from build123d import *

# Parameters (mm, degrees)
SKETCH1_W           = 180
SKETCH1_H           = 165
BOSS_EXTRUDE1_DEPTH = 5
SKETCH2_W           = 4
SKETCH2_H           = 40
CUT_EXTRUDE1_DEPTH  = 5
SKETCH2_3_W         = 4
SKETCH2_3_H         = 35
CUT_EXTRUDE2_DEPTH  = 5
SKETCH3_R           = 1.73
CUT_EXTRUDE3_DEPTH  = 5
SKETCH4_R           = 1.73
CUT_EXTRUDE4_DEPTH  = 5
CUT_EXTRUDE6_DEPTH  = 5
SKETCH5_4_R         = 5.25
SKETCH5_4_W         = 8.6
SKETCH5_4_H         = 14
CUT_EXTRUDE7_DEPTH  = 5
SKETCH6_R           = 1.73
CUT_EXTRUDE8_DEPTH  = 5


with BuildPart() as part:
    # Sketch1 → Boss-Extrude1 (new body)
    with BuildSketch(Plane.XY):
        Rectangle(SKETCH1_W, SKETCH1_H)
    extrude(amount=BOSS_EXTRUDE1_DEPTH)

    # Sketch2 → Cut-Extrude1 (cut)
    with BuildSketch(Plane.XY.offset(5)):
        with Locations((-76, 22.5)):
            Rectangle(SKETCH2_W, SKETCH2_H)
    cut_extrude1 = extrude(amount=-CUT_EXTRUDE1_DEPTH, mode=Mode.SUBTRACT)

    # Sketch2<3> → Cut-Extrude2 (cut)
    with BuildSketch(Plane.XY.offset(5)):
        with Locations((-76, -50)):
            Rectangle(SKETCH2_3_W, SKETCH2_3_H)
    cut_extrude2 = extrude(amount=-CUT_EXTRUDE2_DEPTH, mode=Mode.SUBTRACT)

    # Mirror1: Cut-Extrude1, Cut-Extrude2 across plane
    add(cut_extrude1.mirror(Plane(origin=(0, 0, 0), x_dir=(0, 0, 1), z_dir=(1, 0, 0))), mode=Mode.SUBTRACT)
    add(cut_extrude2.mirror(Plane(origin=(0, 0, 0), x_dir=(0, 0, 1), z_dir=(1, 0, 0))), mode=Mode.SUBTRACT)

    # Sketch3 → Cut-Extrude3 (cut)
    with BuildSketch(Plane(origin=(0, 0, 0), x_dir=(-1, 0, 0), z_dir=(0, 0, -1))):
        with Locations((-84, -77.5)):
            Circle(SKETCH3_R)
        with Locations((-84, -25.5)):
            Circle(SKETCH3_R)
        with Locations((-84, 29.5)):
            Circle(SKETCH3_R)
        with Locations((-84, 64.5)):
            Circle(SKETCH3_R)
    cut_extrude3 = extrude(amount=-CUT_EXTRUDE3_DEPTH, mode=Mode.SUBTRACT)

    # Mirror2: Cut-Extrude3 across plane
    add(cut_extrude3.mirror(Plane(origin=(0, 0, 0), x_dir=(0, 0, 1), z_dir=(1, 0, 0))), mode=Mode.SUBTRACT)

    # Sketch4 → Cut-Extrude4 (cut)
    with BuildSketch(Plane(origin=(0, 0, 0), x_dir=(-1, 0, 0), z_dir=(0, 0, -1))):
        with Locations((-20.24, 52.5)):
            Circle(SKETCH4_R)
        with Locations((20.24, 52.5)):
            Circle(SKETCH4_R)
        with Locations((-27.9, -17.28)):
            Circle(SKETCH4_R)
        with Locations((27.9, -17.28)):
            Circle(SKETCH4_R)
    extrude(amount=-CUT_EXTRUDE4_DEPTH, mode=Mode.SUBTRACT)

    # Sketch5 → Cut-Extrude6 (cut)
    with BuildSketch(Plane(origin=(0, 0, 0), x_dir=(-1, 0, 0), z_dir=(0, 0, -1))):
        Polygon((-56.244150745, 73.117395969), (-61.244150745, 73.117395969), (-61.244150745, 51.117395969), (-51.244150745, 51.117395969), (-51.244150745, 73.117395969), align=None)
    extrude(amount=-CUT_EXTRUDE6_DEPTH, mode=Mode.SUBTRACT)

    # Sketch5<4> → Cut-Extrude7 (cut)
    with BuildSketch(Plane(origin=(0, 0, 0), x_dir=(-1, 0, 0), z_dir=(0, 0, -1))):
        with Locations((59.260446157, 29.480985143)):
            Circle(SKETCH5_4_R)
        with Locations((59.260446157, -13.621859261)):
            Circle(SKETCH5_4_R)
        with Locations((56, 55.117395969)):
            Rectangle(SKETCH5_4_W, SKETCH5_4_H)
    extrude(amount=-CUT_EXTRUDE7_DEPTH, mode=Mode.SUBTRACT)

    # Sketch6 → Cut-Extrude8 (cut)
    with BuildSketch(Plane(origin=(0, 0, 0), x_dir=(-1, 0, 0), z_dir=(0, 0, -1))):
        with Locations((0, -70.5)):
            Circle(SKETCH6_R)
        with Locations((-15, -70.5)):
            Circle(SKETCH6_R)
        with Locations((15, -70.5)):
            Circle(SKETCH6_R)
    extrude(amount=-CUT_EXTRUDE8_DEPTH, mode=Mode.SUBTRACT)


solid = part.part
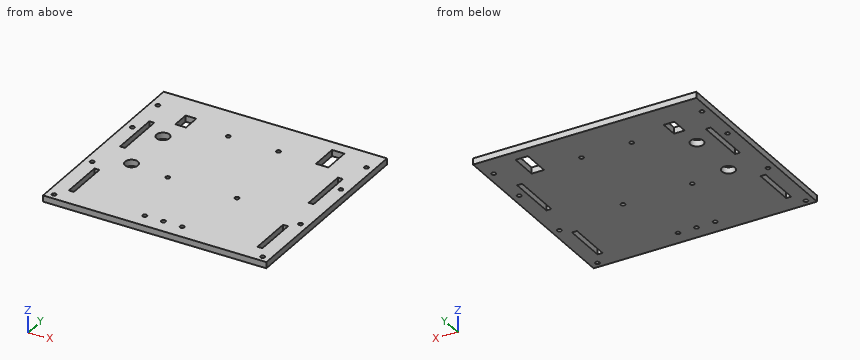
Verification items for the finished model (mm, model axes). Give positions to 0.01 mm unless a question says otherwise; leave off trailing zeros. Loops run counter-clockwise (first coordinate to the right, second up) from the corner with the lowest first, then second, coordinate; pieces in that order, holes last. Notation, with made-up numbers: (7.25, -4.75) - (55.25, -4.75) arc R33 cw to (55.25, 24.25) - close; hole circle Ø9 at (10, 22.25). An arc over 180 degrees is marked (long way). Write item = value, one per line. Start each with the question number.
Q1. Cross-section at C-C, the plane z = 3. State how many separate pieces and enclosed holes the cut face has, and give its area (3 significant figures).
Q2. Cross-section at B-B, the plane y = -37. Enter the section's corners in (x, z), and give its area (3 significant figures).
Q3. Thickness scan on line 1 (X direction, y = 64.5, z = 1.7); line 2 (Y direction, x = -84, z = 2.5); line 3 (X direction, y = 56, z = 1.2). Record the ranges inside material, lowest first.
Q4. Cross-section at A-A, the plane x = 57. Enter the section's corners in (y, z).
Q5. Depth check by flat-ended pin: P1, Ø2, axis at x = -84, y = -25.5, coming from the +Z side. Enter the tip coordinate at first touch or a pass-through.
Answer key:
q1.separate_pieces = 1
q1.enclosed_holes = 23
q1.area = 28,400 mm^2
q2.outline = (-90, 0) - (-78, 0) - (-78, 5) - (-90, 5) - close; (-74, 0) - (74, 0) - (74, 5) - (-74, 5) - close; (78, 0) - (90, 0) - (90, 5) - (78, 5) - close
q2.area = 860 mm^2
q3.line_1 = -90 to -85.73, -82.27 to 51.24, 61.24 to 82.27, 85.73 to 90
q3.line_2 = -82.5 to -79.23, -75.77 to -27.23, -23.77 to 27.77, 31.23 to 62.77, 66.23 to 82.5
q3.line_3 = -90 to -60.3, -51.7 to 51.24, 61.24 to 90
q4.outline = (-82.5, 0) - (51.12, 0) - (51.12, 5) - (-82.5, 5) - close; (73.12, 0) - (82.5, 0) - (82.5, 5) - (73.12, 5) - close
q5.P1 = through
